Build history of the part. All positions in model axes, mm. Face numbers are marked on the shaded views. A direction names the side the tool comes from. Round coordinates to 2 decimals unless told otherwise and drop trailing zeros. Write each loop counter-clockwise with the first axis right and the second up, starting at its lowest first coordinate (ties: lowest second). Pieces come first, ordered by that corner, then holes. Notation, with made-up numbers: (-36.5, -14) -> (-7.5, -14) arc R8 ccw to (-7.5, -7) -> close; hole circle Ø7 at (39.5, 43). An arc over 180 degrees is marked (long way). Answer in a Markdown table with one row per item. Add a question column.
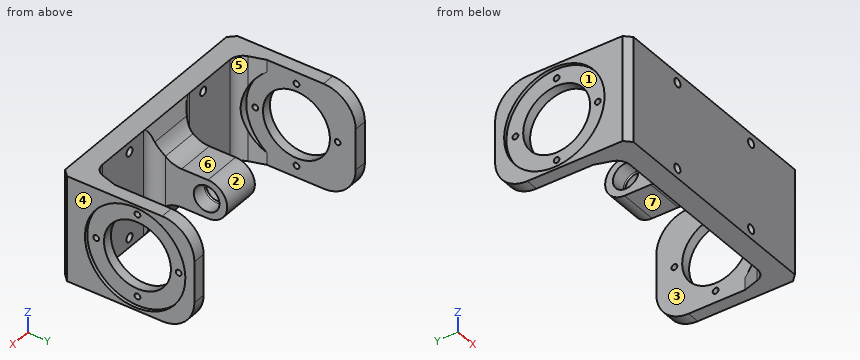
from build123d import *

# Parameters (mm, degrees)
BOSS_EXTRUDE1_DEPTH      = 82
SKETCH5_R                = 10
CUT_EXTRUDE1_DEPTH       = 12
CUT_EXTRUDE2_REACH       = 161.844
SKETCH6_R                = 9
CUT_EXTRUDE4_REACH       = 158.033
SKETCH8_R                = 26
CUT_EXTRUDE5_REACH       = 163.543
FILLET3_R                = 25
SKETCH13_R               = 39
CUT_EXTRUDE6_DEPTH       = 2.5
M4_CLEARANCE_HOLE1_D     = 4.5
M4_CLEARANCE_HOLE1_DEPTH = 7.5
FILLET5_R                = 0.8
CHAMFER1_SIZE            = 5
CHAMFER2_SIZE            = 5
BOSS_EXTRUDE3_START      = -82
BOSS_EXTRUDE3_DEPTH      = 82
SKETCH19_R               = 39
CUT_EXTRUDE7_DEPTH       = 20
M6_CLEARANCE_HOLE1_D     = 6.6
FILLET6_START            = -82.0000001
FILLET6_DEPTH            = 82.0000001
FILLET6_START_2          = -26
FILLET6_2_DEPTH          = 52


with BuildPart() as part:
    # Sketch1 → Boss-Extrude1 (new body)
    with BuildSketch(Plane.XY):
        Polygon((0, 0), (-82.5, 0), (-92.5, 0), (-92.5, 104), (-82.5, 104), (-82.5, 10), (-15, 10), (-15, 74), (0, 74), align=None)
    extrude(amount=-BOSS_EXTRUDE1_DEPTH)

    # Sketch5 → Cut-Extrude1 (cut)
    with BuildSketch(Plane.ZY.offset(15)):
        with Locations(Location((-41, 58, 0), (0, 0, 270))):
            Circle(SKETCH5_R)
    extrude(amount=-CUT_EXTRUDE1_DEPTH, mode=Mode.SUBTRACT)

    # Sketch6 → Cut-Extrude2 (cut, up to next)
    with BuildSketch(Plane.ZY.offset(3), mode=Mode.PRIVATE) as cut_extrude2_sk1:
        with Locations(Location((-41, 58, 0), (0, 0, 270))):
            Circle(SKETCH6_R)
    cut_extrude2_tool1 = extrude(cut_extrude2_sk1.sketch, amount=-CUT_EXTRUDE2_REACH, mode=Mode.PRIVATE) & part.part
    add(cut_extrude2_tool1.solids().sort_by_distance((-3, 58, -41))[0], mode=Mode.SUBTRACT)

    # Sketch8 → Cut-Extrude4 (cut, up to next)
    with BuildSketch(Plane(origin=(-82.5, 0, 0), x_dir=(0, 0, -1), z_dir=(1, 0, 0)), mode=Mode.PRIVATE) as cut_extrude4_sk1:
        with Locations(Location((41, 58, 0), (0, 0, 90))):
            Circle(SKETCH8_R)
    cut_extrude4_tool1 = extrude(cut_extrude4_sk1.sketch, amount=-CUT_EXTRUDE4_REACH, mode=Mode.PRIVATE) & part.part
    add(cut_extrude4_tool1.solids().sort_by_distance((-82.5, 58, -41))[0], mode=Mode.SUBTRACT)

    # Sketch10 → Cut-Extrude5 (cut, up to next)
    with BuildSketch(Plane(origin=(0, 0, 0), x_dir=(0, 0, -1), z_dir=(1, 0, 0)), mode=Mode.PRIVATE) as cut_extrude5_sk1:
        with BuildLine():
            Line((0, 74), (0, 16))
            Line((0, 16), (11.714285714, 19.492525222))
            ThreePointArc((11.714285714, 19.492525222), (22.035674515, 26.706536079), (26, 38.658822172))
            Line((26, 38.658822172), (26, 59))
            ThreePointArc((26, 59), (30.393398282, 69.606601718), (41, 74))
            Line((41, 74), (0, 74))
        make_face()
    cut_extrude5_tool1 = extrude(cut_extrude5_sk1.sketch, amount=-CUT_EXTRUDE5_REACH, mode=Mode.PRIVATE) & part.part
    # Sketch10 → Cut-Extrude5 (cut, up to next)
    with BuildSketch(Plane(origin=(0, 0, 0), x_dir=(0, 0, -1), z_dir=(1, 0, 0)), mode=Mode.PRIVATE) as cut_extrude5_sk2:
        with BuildLine():
            Line((82, 74), (41, 74))
            ThreePointArc((41, 74), (51.606601718, 69.606601718), (56, 59))
            Line((56, 59), (56, 38.658822172))
            ThreePointArc((56, 38.658822172), (59.964325485, 26.706536079), (70.285714286, 19.492525222))
            Line((70.285714286, 19.492525222), (82, 16))
            Line((82, 16), (82, 74))
        make_face()
    cut_extrude5_tool2 = extrude(cut_extrude5_sk2.sketch, amount=-CUT_EXTRUDE5_REACH, mode=Mode.PRIVATE) & part.part
    add(cut_extrude5_tool1.solids().sort_by_distance((0, 48.321716, -12.955067))[0], mode=Mode.SUBTRACT)
    add(cut_extrude5_tool2.solids().sort_by_distance((0, 48.321716, -69.044933))[0], mode=Mode.SUBTRACT)

    # Fillet3
    fillet3_edges = [part.edges().sort_by_distance(p)[0] for p in [
        (-87.5, 104, 0),
        (-87.5, 104, -82),
    ]]
    fillet(fillet3_edges, radius=FILLET3_R)

    # Sketch13 → Cut-Extrude6 (cut)
    with BuildSketch(Plane.ZY.offset(92.5)):
        with Locations((-41, 58)):
            Circle(SKETCH13_R)
    extrude(amount=-CUT_EXTRUDE6_DEPTH, mode=Mode.SUBTRACT)

    # M4 Clearance Hole1
    with Locations(Plane.ZY.offset(90)):
        with Locations((-41, 90), (-9, 58), (-41, 26), (-73, 58)):
            Hole(M4_CLEARANCE_HOLE1_D / 2, depth=M4_CLEARANCE_HOLE1_DEPTH)

    # Fillet5
    fillet5_edges = [part.edges().sort_by_distance(p)[0] for p in [
        (-3, 68, -41),
    ]]
    fillet(fillet5_edges, radius=FILLET5_R)

    # Mirror1: part across plane


with BuildPart() as part_1:
    add(part.part)
    add(part.part.mirror(Plane(origin=(0, 74, -82), x_dir=(0, 0, 1), z_dir=(1, 0, 0))))

    # Chamfer1
    chamfer1_edges = [part_1.edges().sort_by_distance(p)[0] for p in [
        (92.5, 0, -41),
        (-92.5, 0, -41),
    ]]
    chamfer(chamfer1_edges, length=CHAMFER1_SIZE)

    # Chamfer2
    chamfer2_edges = [part_1.edges().sort_by_distance(p)[0] for p in [
        (82.5, 10, -41),
        (-82.5, 10, -41),
    ]]
    chamfer(chamfer2_edges, length=CHAMFER2_SIZE)

    # Sketch18 → Boss-Extrude3 (add)
    with BuildSketch(Plane.XY.offset(BOSS_EXTRUDE3_START)):
        with BuildLine():
            Line((-82.5, 35), (-78.726174588, 23))
            ThreePointArc((-78.726174588, 23), (-75.102862357, 17.937742252), (-69.186782574, 16))
            Line((-69.186782574, 16), (0, 16))
            Line((0, 16), (0, 10))
            Line((0, 10), (-77.5, 10))
            Line((-77.5, 10), (-82.5, 15))
            Line((-82.5, 15), (-82.5, 35))
        make_face()
    boss_extrude3 = extrude(amount=BOSS_EXTRUDE3_DEPTH)

    # Mirror2: Boss-Extrude3 across plane
    add(boss_extrude3.mirror(Plane(origin=(0, 0, 0), x_dir=(0, 0, 1), z_dir=(1, 0, 0))))

    # Sketch19 → Cut-Extrude7 (cut)
    with BuildSketch(Plane(origin=(-82.5, 0, 0), x_dir=(0, 0, -1), z_dir=(1, 0, 0))):
        with Locations(Location((41, 58, 0), (0, 0, 180))):
            Circle(SKETCH19_R)
    cut_extrude7 = extrude(amount=CUT_EXTRUDE7_DEPTH, mode=Mode.SUBTRACT)

    # Mirror3: Cut-Extrude7 across plane
    add(cut_extrude7.mirror(Plane(origin=(0, 0, 0), x_dir=(0, 0, 1), z_dir=(1, 0, 0))), mode=Mode.SUBTRACT)

    # M6 Clearance Hole1 (through all)
    with Locations(Plane(origin=(0, 0, 0), x_dir=(-1, 0, 0), z_dir=(0, -1, 0))):
        with Locations((-40, 74.5), (40, 74.5), (40, 7.5), (-40, 7.5)):
            Hole(M6_CLEARANCE_HOLE1_D / 2)

    # Fillet6: read off the stored shape, not the designer's step
    # Fillet6 outline → Fillet6 (add)
    with BuildSketch(Plane.XY.offset(FILLET6_START)):
        with BuildLine():
            Line((15, 16), (25, 16))
            ThreePointArc((25, 16), (17.928932188, 18.928932188), (15, 26))
            Line((15, 26), (15, 16))
        make_face()
        with BuildLine():
            ThreePointArc((-15, 26), (-17.928932188, 18.928932188), (-25, 16))
            Line((-25, 16), (-15, 16))
            Line((-15, 16), (-15, 26))
        make_face()
    extrude(amount=FILLET6_DEPTH)

    # Fillet6 2 outline → Fillet6 2 (cut)
    with BuildSketch(Plane.YZ.offset(FILLET6_START_2)):
        with BuildLine():
            Line((19.492525222, -70.285714286), (16, -82))
            Line((16, -82), (26, -82.0000001))
            Line((26, -82.0000001), (26, -60.516001123))
            ThreePointArc((26, -60.516001123), (22.013361061, -64.912681821), (19.492525222, -70.285714286))
        make_face()
        with BuildLine():
            Line((26, 0), (16, 0))
            Line((16, 0), (19.492525222, -11.714285714))
            ThreePointArc((19.492525222, -11.714285714), (22.013361061, -17.087318179), (26, -21.483998877))
            Line((26, -21.483998877), (26, 0))
        make_face()
    extrude(amount=FILLET6_2_DEPTH, mode=Mode.SUBTRACT)


solid = part_1.part
(1) Saw through at C-C (z = -41). Count the separate pieces of the cut face and the enclosed holes in it, plus the area to 3 significant figures.
(2) Which spindle directions (+Z, -Z, +X, -X, +Y, -Y) get a long thin tool onto all of the face, cutting with end or side? Do the marked faces 5, 6 and 7. Say none if no direction does.
(3) Probe line 1 along X through (y, z) = (95, -35); line 2 along X through (y, z) = (97, -65); line 3 along Y through (x, z) = (-87.75, -41). List the from-to ranges inside material, lowest first.
(4) Saw through at D-D (x = 47). List the corners of the cut face in (y, z).
(5) Mould opens along Z. For the marked faces 1, 2, 3 and 4 say: pulls with the +Z half, pulls with the -Z half, needs draft (parallel to the pull), parting line crosses it, or undercut.
(6) Drop flat-ended pins along their axis: P1, Ø5, axis at x = 8.5, z = -46.5, coming from the +Y side; P2, Ø13.5, axis at x = -51.5, z = -39, coming from the +Y side; P3, Ø5, axis at x = 14.5, z = -48, coming from the +Y side. Give the stop position or say it passes through.
(7) Saw through at A-A (x = -6.5). List the corners of the cut face in (y, z).
(8) Saw through at B-B (y = 90). List the corners of the cut face in (x, z).
Answer sheet:
| question | item | result |
|---|---|---|
| 1 | separate pieces | 8 |
| 1 | enclosed holes | 0 |
| 1 | area | 4,640 mm² |
| 2 | face 5 | +Z, -Z, +Y |
| 2 | face 6 | +Z, +X, -X, +Y |
| 2 | face 7 | -Z, +X, -X, +Y |
| 3 | line 1 | x = -90 to -82.5, 82.5 to 90 |
| 3 | line 2 | x = -92.5 to -82.5, 82.5 to 92.5 |
| 3 | line 3 | y = 0.25 to 23.75, 28.25 to 32, 84 to 87.75, 92.25 to 104 |
| 4 | outline | (0, -82) -> (16, -82) -> (16, 0) -> (0, 0) -> close |
| 5 | face 1 | undercut |
| 5 | face 2 | parting line crosses it |
| 5 | face 3 | undercut |
| 5 | face 4 | needs draft |
| 6 | P1 | stops at y = 73.7 |
| 6 | P2 | stops at y = 16 |
| 6 | P3 | stops at y = 73.31 |
| 7 | outline | (0, -82) -> (16, -82) -> (19.49, -70.29) arc R20 cw to (38.66, -56) -> (59, -56) arc R15 ccw to (59, -26) -> (38.66, -26) arc R20 cw to (19.49, -11.71) -> (16, 0) -> (0, 0) -> close; hole circle Ø20 at (58, -41) |
| 8 | outline | (-92.5, -79.45) -> (-82.5, -79.45) -> (-82.5, -43.25) -> (-90, -43.25) -> (-90, -63.29) -> (-92.5, -63.29) -> close; (-92.5, -18.71) -> (-90, -18.71) -> (-90, -38.75) -> (-82.5, -38.75) -> (-82.5, -2.55) -> (-92.5, -2.55) -> close; (82.5, -79.45) -> (92.5, -79.45) -> (92.5, -63.29) -> (90, -63.29) -> (90, -43.25) -> (82.5, -43.25) -> close; (82.5, -38.75) -> (90, -38.75) -> (90, -18.71) -> (92.5, -18.71) -> (92.5, -2.55) -> (82.5, -2.55) -> close |
